Could you check a few things on this model? Use its own coordinates, in mm. A direction names the side the tool comes from. Round coordinates to 2 decimals unless told otherwise and drop trailing zeros. Write each loop counter-clockwise with the first axis right and the second up, starting at its lowest first coordinate (ties: lowest second). Pieces come first, ordered by that corner, then holes. Notation, with made-up numbers: (71, 28) - (112, 28) arc R18 cw to (112, 57) - close; hole circle Ø3 at (69.5, -38.5). An arc over 180 degrees is marked (long way). Put each result on its own line as item: value.
Solid Edge part; units mm, degrees
sketch "Sketch1" plane through (0, 0, 0) normal (0, -1, 0) x (1, 0, 0)
  circle A0 centre (0, 0) radius 11
  circle A1 centre (8, 0) radius 1.75
  circle A2 centre (0, -7.9975) radius 1.75
  circle A3 centre (-8, 0) radius 1.75
  circle A4 centre (0, 8) radius 1.75
  circle A5 centre (0, 0) radius 4
extrude "Protrusion1" add sketch "Sketch1" against normal blind 3.5
sketch "Sketch2" plane through (0, 0, 0) normal (0, -1, 0) x (1, 0, 0)
  circle A0 centre (0, 0) radius 4
  circle A1 centre (0, 0) radius 4.5
extrude "ExtrudedProtrusion_2" add sketch "Sketch2" along normal blind 1.5
chamfer "Chamfer_1" distance 0.3 angle 45 1 edges at (-4.5, -1.5, 0)
chamfer "Chamfer_2" distance 0.3 angle 45 2 edges at (-11, 0, 0) (-11, 3.5, 0)
sketch "Sketch3" plane through (0, 3.5, 0) normal (0, 1, 0) x (0, 0, -1)
  circle A0 centre (0, 0) radius 4.5
  circle A1 centre (0, 0) radius 4
extrude "ExtrudedProtrusion_3" add sketch "Sketch3" along normal blind 10
properties material "Brass, yellow brass"
(1) Please list where these lines run through material, in increasing order: probe 1 along Z at (x, y) = (0, 2.35); probe 2 along Y at (x, z) = (4.5, 1.25); probe 3 along X at (y, z) = (5.75, -2.5). Write a range as from..to.
Values found:
probe 1: z = -11..-9.75, -6.25..-4, 4..6.25, 9.75..11
probe 2: y = 0..3.5
probe 3: x = -3.74..-3.12, 3.12..3.74
(2) Imagine slicing it at A-A, the plane z = 0. Give the number of separate pieces and of enclosed holes in the cut face, then the cut area to 3 significant figures.
Values found:
separate pieces: 4
enclosed holes: 0
area: 35.7 mm^2
(3) If we mould it in two halves opening along Z, with no side actions, what happens to faces 1 (the face through (-2.38, 1.73, -10.74)), 2 (the face through (-6.331, 1.726, 0.526)), 3 (the face through (0, 0, -5))? For each: pulls with the +Z half, pulls with the -Z half, needs draft (parallel to the pull), parting line crosses it, or undercut.
Values found:
face 1: parting line crosses it
face 2: undercut
face 3: needs draft
(4) I'm going to push flat-ended pins straight in: pin 1 (4 mm diameter, centred on x = -8, z = 0, fed in from -Y); pin 2 (8 mm diameter, centred on y = 12, z = -3.5, fed in from -X); pin 3 (3 mm diameter, centred on x = 5, y = 9, fed in from -Z). Where does each tip first touch, or does it pass through?
Values found:
pin 1: stops at y = 0
pin 2: stops at x = -4.5
pin 3: stops at z = -2.83
(5) For faces 4 (the face through (4.46, 8.43, 0.59)), 5 (the face through (1.49, 5.9, -3.71)), 6 (the face through (-0.59, -0.59, -4.46)), which set-ups out of +Z, -Z, +X, -X, +Y, -Y let a thin tool reach every point of the face, with its end or its side?
Values found:
face 4: +Y
face 5: +Y, -Y
face 6: -Y
(6) Imagine slicing it at C-C, the plane y = 7.5. List the corners of the cut face in (x, z) for me, then the cut area to 3 significant figures.
Values found:
outline: circle Ø9 at (0, 0); hole circle Ø8 at (0, 0)
area: 13.4 mm^2
